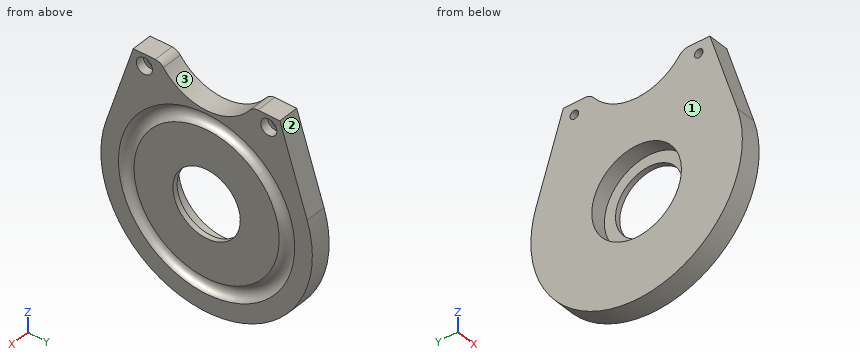
from build123d import *

# Parameters (mm, degrees)
EXTRUDE_1_DEPTH     = 8
SKETCH_4_R          = 3.105
CUT_EXTRUDE_1_DEPTH = 3.3
SKETCH_5_R          = 1.65
CUT_EXTRUDE_2_DEPTH = 61.923969011
SKETCH_6_R          = 17.3
CUT_EXTRUDE_3_DEPTH = 6
SKETCH_7_R          = 13
CUT_EXTRUDE_4_DEPTH = 62.038020938


with BuildPart() as part:
    # 草图1 → 凸台-拉伸1 (new body)
    with BuildSketch(Plane(origin=(0, 0, 0), x_dir=(0, 0, -1), z_dir=(1, 0, 0))):
        with BuildLine():
            Line((-45, -19.810035336), (-45, -28.278272418))
            Line((-45, -28.278272418), (-12.60789337, -38.803105865))
            ThreePointArc((-12.60789337, -38.803105865), (40.8, 0), (-12.60789337, 38.803105865))
            Line((-12.60789337, 38.803105865), (-45, 28.278272418))
            Line((-45, 28.278272418), (-45, 19.810035336))
            ThreePointArc((-45, 19.810035336), (-44.588871689, 18.043683162), (-43.44, 16.640429682))
            ThreePointArc((-43.44, 16.640429682), (-35.25, 0), (-43.44, -16.640429682))
            ThreePointArc((-43.44, -16.640429682), (-44.588871689, -18.043683162), (-45, -19.810035336))
        make_face()
    extrude(amount=EXTRUDE_1_DEPTH)

    # 草图3 → 切除-旋转1 (revolve, cut)
    with BuildSketch(Plane(origin=(0, 0, 0), x_dir=(1, 0, 0), z_dir=(0, 1, 0)), mode=Mode.PRIVATE) as cut_revolve_1_sk:
        with BuildLine():
            Line((8, 34), (8, 28))
            ThreePointArc((8, 28), (5, 31), (8, 34))
        make_face()
    revolve(cut_revolve_1_sk.sketch.rotate(Axis((0, 0, 0), (1, 0, 0)), 180), axis=Axis((0, 0, 0), (1, 0, 0)), mode=Mode.SUBTRACT)

    # 草图4 → 切除-拉伸1 (cut)
    with BuildSketch(Plane(origin=(8, 0, 0), x_dir=(0, 0, -1), z_dir=(1, 0, 0))):
        with Locations((-40.5, -23.998774784)):
            Circle(SKETCH_4_R)
        with Locations(Location((-40.5, 23.998774784, 0), (0, 0, 180))):
            Circle(SKETCH_4_R)
    extrude(amount=-CUT_EXTRUDE_1_DEPTH, mode=Mode.SUBTRACT)

    # 草图5 → 切除-拉伸2 (cut, through all)
    with BuildSketch(Plane(origin=(4.7, 0, 0), x_dir=(0, 0, -1), z_dir=(1, 0, 0))):
        with Locations((-40.5, -23.998774784)):
            Circle(SKETCH_5_R)
        with Locations(Location((-40.5, 23.998774784, 0), (0, 0, 180))):
            Circle(SKETCH_5_R)
    extrude(amount=-CUT_EXTRUDE_2_DEPTH, mode=Mode.SUBTRACT)

    # 草图6 → 切除-拉伸3 (cut)
    with BuildSketch(Plane.ZY):
        Circle(SKETCH_6_R)
    extrude(amount=-CUT_EXTRUDE_3_DEPTH, mode=Mode.SUBTRACT)

    # 草图7 → 切除-拉伸4 (cut, through all)
    with BuildSketch(Plane.ZY.offset(-6)):
        Circle(SKETCH_7_R)
    extrude(amount=-CUT_EXTRUDE_4_DEPTH, mode=Mode.SUBTRACT)


solid = part.part
Read the model definition and answer for the solid it produces. Units are mm, in the model's axes. Face numbers are marked on the shaded views. Give positions to 0.01 mm unless a question says otherwise; leave off trailing zeros. Write each loop counter-clockwise with the first axis right and the second up, starting at its lowest first coordinate (ties: lowest second). Pieces come first, ordered by that corner, then holes. Notation, with made-up numbers: M 64.25,62.5 L 115.25,62.5 A15 ccw 115.25,68.5 Z; hole C 31.5,41.5 d8. An arc over 180 degrees is marked long. One line per item, written item: value. Start each with the question number.
(1) Find section B-B (z = 0). Determine the outline of the cut face in (x, y), plus the area to 3 significant figures.
(2) Flat-ended cylindrical pins translate along their axes: pin 1 Ø2 at (y, z) = (-24, 40.5) entering from -X (3 decimals); pin 2 Ø4 at (y, z) = (24, 40.5) entering from +X; pin 3 Ø4 at (x, y) = (2.5, -28) entering from -Z. Find the tip coordinate at first contact, or state that the pin passes through.
(3) Find the intervals of material crossed by line 1 (Z direction, x = 6.5, y = -14); line 2 (Y direction, x = 7.55, z = 0); line 3 (Y direction, x = 1.95, z = 0), in increasing order.
(4) Find section D-D (z = 40.5). Determine the outline of the cut face in (x, y), plus the area to 3 significant figures.
(5) Find section C-C (x = 3.25). Determine the outline of the cut face in (y, z), plus the area to 3 significant figures.
(6) Determine the mould class of the marked faces 1, 2 and 3 for opening direction Y: pulls with the +Y half, pulls with the -Y half, needs draft (parallel to the pull), parting line crosses it, or undercut.
(7) Find section A-A (y = 0). Determine the outline of the cut face in (x, z), plus the area to 3 significant figures.
Results below:
1. outline: M 0,-40.8 L 8,-40.8 L 8,-34 A3 cw 8,-28 L 8,-13 L 6,-13 L 6,-17.3 L 0,-17.3 Z; M 0,17.3 L 6,17.3 L 6,13 L 8,13 L 8,28 A3 cw 8,34 L 8,40.8 L 0,40.8 Z
1. area: 365 mm^2
2. pin 1: passes through
2. pin 2: stops at x = 4.7
2. pin 3: stops at z = -31.44
3. line 1: z = -38.32 to -30.54, -24.71 to 24.71, 30.54 to 40.6
3. line 2: y = -40.8 to -33.97, -28.03 to -13, 13 to 28.03, 33.97 to 40.8
3. line 3: y = -40.8 to -17.3, 17.3 to 40.8
4. outline: M 0,-29.74 L 8,-29.74 L 8,-27.1 L 4.7,-27.1 L 4.7,-25.65 L 0,-25.65 Z; M 0,-22.35 L 4.7,-22.35 L 4.7,-20.89 L 8,-20.89 L 8,-13.89 L 0,-13.89 Z; M 0,13.89 L 8,13.89 L 8,20.89 L 4.7,20.89 L 4.7,22.35 L 0,22.35 Z; M 0,25.65 L 4.7,25.65 L 4.7,27.1 L 8,27.1 L 8,29.74 L 0,29.74 Z
4. area: 182 mm^2
5. outline: M -38.8,12.61 A40.8 ccw long 38.8,12.61 L 28.28,45 L 19.81,45 A4 ccw 16.64,43.44 A21 cw -16.64,43.44 A4 ccw -19.81,45 L -28.28,45 Z; hole C -24,40.5 d3.3; hole C 0,0 d34.6; hole C 24,40.5 d3.3
5. area: 4,600 mm^2
6. face 1: needs draft
6. face 2: pulls with the +Y half
6. face 3: undercut
7. outline: M 0,-40.8 L 8,-40.8 L 8,-34 A3 cw 8,-28 L 8,-13 L 6,-13 L 6,-17.3 L 0,-17.3 Z; M 0,17.3 L 6,17.3 L 6,13 L 8,13 L 8,28 A3 cw 8,34 L 8,35.25 L 0,35.25 Z
7. area: 321 mm^2
